Read the model definition and answer for the solid it produces. Units are mm, in the model's axes. Face numbers are marked on the shaded views. A direction names the side the tool comes from. Give positions to 0.01 mm unless a question says otherwise; leave off trailing zeros. Write each loop counter-clockwise with the first axis right and the second up, starting at its lowest first coordinate (ties: lowest second). Pieces come first, ordered by that corner, then holes. Notation, with made-up numbers: (-9.5, 60.25) -> (-2.5, 60.25) arc R38 cw to (-2.5, 98.25) -> close; hole circle Ø4 at (-32.75, 26). An arc over 180 degrees is marked (long way). Write item = value, one per line.
from build123d import *

# Parameters (mm, degrees)
CYLINDER019_R                      = 2.5
CYLINDER019_DEPTH                  = 25
CYLINDER018_R                      = 4.36
CYLINDER018_DEPTH                  = 5
FUSION001018017020_PLACEMENT_ANGLE = 180
POCKET002018004005_DEPTH           = 2.5


with BuildPart() as cylinder019:
    # Cylinder019 → Cylinder019 (new body)
    with BuildSketch(Plane.XY):
        Circle(CYLINDER019_R)
    extrude(amount=CYLINDER019_DEPTH)


with BuildPart() as obj1:
    # Cylinder018 → Cylinder018 (new body)
    with BuildSketch(Plane.XY):
        Circle(CYLINDER018_R)
    extrude(amount=CYLINDER018_DEPTH)

    # Fusion001018017020: union Cylinder019
    add(cylinder019.part)


with BuildPart() as obj1_1:
    # Fusion001018017020 placement: moved
    add(obj1.part.rotate(Axis((0, 0, 0), (0, 1, 0)), FUSION001018017020_PLACEMENT_ANGLE))

    # Sketch022 → Pocket002018004005 (cut)
    with BuildSketch(Plane(origin=(0, 0, 0), x_dir=(-1, 0, 0), z_dir=(0, 0, 1))):
        Polygon((2, -1.154701), (2, 1.154701), (0, 2.309401), (-2, 1.154701), (-2, -1.154701), (0, -2.309401), align=None)
    extrude(amount=-POCKET002018004005_DEPTH, mode=Mode.SUBTRACT)


solid = obj1_1.part
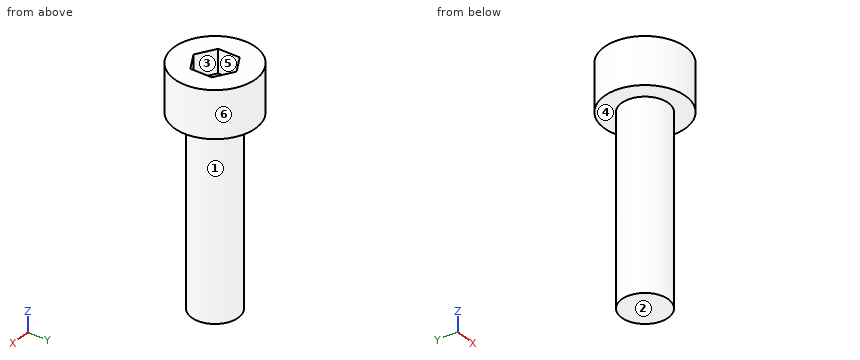
(1) The part is cut by section B-B on z = -16.75. Determine the outline of the cut face in (x, y).
Checks:
outline = circle Ø5 at (0, 0)
(2) The part is cut by section D-D on y = -2.75. Determine the outline of the cut face in (x, z), plus the area to 3 significant figures.
Checks:
outline = (-3.38, -5) -> (3.38, -5) -> (3.38, 0) -> (-3.38, 0) -> close
area = 33.8 mm²
(3) The part is cut by section C-C on x = -1. Determine the outline of the cut face in (y, z).
Checks:
outline = (-4.24, -5) -> (-2.29, -5) -> (-2.29, -25) -> (2.29, -25) -> (2.29, -5) -> (4.24, -5) -> (4.24, 0) -> (1.73, 0) -> (1.73, -2.5) -> (-1.73, -2.5) -> (-1.73, 0) -> (-4.24, 0) -> close
(4) A tool of negligible diameter and unlimited length cuts with its end or side. For the marked faces 4, 5 and 6, from which of +Z, -Z, +X, -X, +Y, -Y can it reach the whole face along a straight path? Write none if from no direction.
Checks:
face_4 = -Z
face_5 = +Z
face_6 = +Z, -Z
(5) Consider L1, parallel to Z at x = 2, y = -2.75; L2, parallel to X at y = 1.5, z = -9.75; L3, parallel to X at y = 0, z = -20.75. Determine where each line is inside the solid, lowest interval first.
Checks:
L1 = -5 to 0
L2 = -2 to 2
L3 = -2.5 to 2.5
(6) The part is cut by section A-A on y = 0. Determine the outline of the cut face in (x, z), plus the area to 3 significant figures.
Checks:
outline = (-4.36, -5) -> (-2.5, -5) -> (-2.5, -25) -> (2.5, -25) -> (2.5, -5) -> (4.36, -5) -> (4.36, 0) -> (2, 0) -> (2, -2.5) -> (-2, -2.5) -> (-2, 0) -> (-4.36, 0) -> close
area = 134 mm²
(7) For a pull along Y with two mould halves and no side action, classify the marked faces 1, 2 and 3 as released by +Y, released by -Y, zero draft, split by the parting line, or undercut.
Checks:
face_1 = split by the parting line
face_2 = zero draft
face_3 = undercut
(8) Given P1, Ø3, axis at y = -1.5, z = -12.5, coming from the +X side; P2, Ø1.5, axis at y = -2.5, z = -5.5, coming from the +X side; P3, Ø1.5, axis at x = 3, z = -18.5, coming from the +Y side, each flat-ended and moving along its own axis, determine where each tip first touches the part or whether it passes through.
Checks:
P1 = 2.5
P2 = 3.9
P3 = 1.09
